```python
from build123d import *

# Parameters (mm, degrees)
MAINBODYS_R    = 4
MAINBODY_DEPTH = 104
HEADS_W        = 7.5
HEADS_H        = 3
HEADFILLET_R   = 0.1


with BuildPart() as part:
    # MainBodyS → MainBody (new body)
    with BuildSketch(Plane(origin=(0, 0, 0), x_dir=(1, 0, 0), z_dir=(0, 1, 0))):
        Circle(MAINBODYS_R)
    extrude(amount=-MAINBODY_DEPTH)

    # HeadS → Head (revolve)
    with BuildSketch(Plane.XY):
        with Locations((3.75, 1.5)):
            Rectangle(HEADS_W, HEADS_H)
    revolve(axis=Axis((0, 0, 0), (0, 1, 0)))

    # HeadIndentS → HeadIndent (revolve, cut)
    with BuildSketch(Plane.XY):
        with BuildLine():
            Line((4, 0), (4, 0.4))
            ThreePointArc((4, 0.4), (4.029289322, 0.470710678), (4.1, 0.5))
            Line((4.1, 0.5), (6, 0.5))
            ThreePointArc((6, 0.5), (6.023974846, 0.497083504), (6.046551241, 0.488504135))
            Line((6.046551241, 0.488504135), (6.953448759, 0.011495865))
            ThreePointArc((6.953448759, 0.011495865), (6.976025154, 0.002916496), (7, 0))
            Line((7, 0), (4, 0))
        make_face()
    revolve(axis=Axis((0, 0, 0), (0, 1, 0)), mode=Mode.SUBTRACT)

    # BottomTipS → BottomTip (revolve)
    with BuildSketch(Plane.XY):
        Polygon((4, -104), (3.5, -105.5), (3.5, -107), (0, -107), (0, -104), align=None)
    revolve(axis=Axis((0, -107, 0), (0, 1, 0)))

    # HeadFillet
    headfillet_edges = [part.edges().sort_by_distance(p)[0] for p in [
        (-7.5, 0, 0),
        (-7.5, 3, 0),
    ]]
    fillet(headfillet_edges, radius=HEADFILLET_R)


solid = part.part
```
CAD build for the part. Positions are in the model's coordinates, mm. A direction names the side the tool comes from. Give positions to 0.01 mm unless a question says otherwise; leave off trailing zeros. Order: outer loops, then holes, each group sorted by start corner. A loop starts at its lowest first (then second) coordinate and runs counter-clockwise, first axis right, second up. Notation, with made-up numbers: M 69,4 L 111,4 A24 cw 111,34 Z; hole C 75,2.25 d10. An arc over 180 degrees is marked long. Put each result on its own line as item: value. Start each with the question number.
(1) Saw through at A-A, the plane z = 0. Write the cut outline in (x, y).
(2) Saw through at B-B, the plane x = 0. Write the cut outline in (y, z), then the cut area to 3 significant figures.
(3) Saw through at C-C, the plane y = -16. Write the cut outline in (x, z).
(4) Which spindle directions (+Z, -Z, +X, -X, +Y, -Y) get a long thin tool onto all of the face, cutting with end or side? Do faces 4 (the flat face through (0, 3, 0)), 5 (the cylindrical face through (-0.867, -51.069, 3.905)). Say none if no direction does.
(5) Flat gauge pins, fed straight in: pin 1 Ø3 at (y, z) = (-51.5, 3) entering from -X; pin 2 Ø3 at (x, z) = (-0.5, -3.5) entering from -Y; pin 3 Ø1 at (x, y) = (4, -33.5) entering from +Z; pin 4 Ø5 at (x, y) = (4.5, -9.5) entering from -Z. Where does each tip first touch, or does it go through?
(6) Drill centre lines: line 1 along Y through (x, z) = (-1.25, -4.5); line 2 along Y through (x, z) = (6, 3.75); line 3 along X through (y, z) = (-50, 0.5). Where is each one in solid material? Low to high.
(7) Mould opens along X. For faces 1 (the cylindrical face through (-7.493, 1.52, -0.33)), 2 (the flat face through (0, -107, 0)), 3 (the flat face through (-3, 0.5, 4)) say: +X half, -X half, draft (parallel to the pull), parting line (faces both ways), or undercut.
Check result:
1. outline: M -7.5,0.1 A0.1 ccw -7.4,0 L -7,0 A0.1 ccw -6.95,0.01 L -6.05,0.49 A0.1 cw -6,0.5 L -4.1,0.5 A0.1 cw -4,0.4 L -4,-104 L -3.5,-105.5 L -3.5,-107 L 3.5,-107 L 3.5,-105.5 L 4,-104 L 4,0.4 A0.1 cw 4.1,0.5 L 6,0.5 A0.1 cw 6.05,0.49 L 6.95,0.01 A0.1 ccw 7,0 L 7.4,0 A0.1 ccw 7.5,0.1 L 7.5,2.9 A0.1 ccw 7.4,3 L -7.4,3 A0.1 ccw -7.5,2.9 Z
2. outline: M -107,-3.5 L -105.5,-3.5 L -104,-4 L 0.4,-4 A0.1 cw 0.5,-4.1 L 0.5,-6 A0.1 cw 0.49,-6.05 L 0.01,-6.95 A0.1 ccw 0,-7 L 0,-7.4 A0.1 ccw 0.1,-7.5 L 2.9,-7.5 A0.1 ccw 3,-7.4 L 3,7.4 A0.1 ccw 2.9,7.5 L 0.1,7.5 A0.1 ccw 0,7.4 L 0,7 A0.1 ccw 0.01,6.95 L 0.49,6.05 A0.1 cw 0.5,6 L 0.5,4.1 A0.1 cw 0.4,4 L -104,4 L -105.5,3.5 L -107,3.5 Z
2. area: 896 mm2
3. outline: C 0,0 d8
4. face 4: +Z, -Z, +X, -X, +Y
4. face 5: -Y
5. pin 1: stops at x = -3.71
5. pin 2: stops at y = -107
5. pin 3: stops at z = 1.94
5. pin 4: stops at z = -3.46
6. line 1: y = 0.5 to 3
6. line 2: y = 0 to 3
6. line 3: x = -3.97 to 3.97
7. face 1: parting line
7. face 2: draft
7. face 3: undercut
